Here's how the part is built. I have some questions about the finished solid (model axes, mm). Face numbers are marked on the shaded views. A direction names the side the tool comes from. Coordinates: 2 decimals unless noted, no trailing zeros. Order: outer loops, then holes, each group sorted by start corner. A loop starts at its lowest first (then second) coordinate and runs counter-clockwise, first axis right, second up.
```python
from build123d import *

# Parameters (mm, degrees)
BOSS_EXTRUDE1_DEPTH = 10
SKETCH2_R           = 1.75
CUT_EXTRUDE1_DEPTH  = 10
BOSS_EXTRUDE2_DEPTH = 5
CUT_EXTRUDE2_DEPTH  = 3
FILLET1_R           = 4
FILLET2_R           = 1.5
FILLET3_R           = 2
FILLET4_R           = 1


with BuildPart() as part:
    # Sketch1 → Boss-Extrude1 (new body)
    with BuildSketch(Plane(origin=(0, 0, 0), x_dir=(1, 0, 0), z_dir=(0, 1, 0))):
        with BuildLine():
            Line((-47.236109069, 5), (-55.236109069, 5))
            Line((-55.236109069, 5), (-55.236109069, -5))
            Line((-55.236109069, -5), (-47.236109069, -5))
            ThreePointArc((-47.236109069, -5), (-47.5, 0), (-47.236109069, 5))
        make_face()
    extrude(amount=-BOSS_EXTRUDE1_DEPTH)

    # Sketch2 → Cut-Extrude1 (cut)
    with BuildSketch(Plane.ZY.offset(55.236109069)):
        with Locations((0, -5)):
            Circle(SKETCH2_R)
    extrude(amount=-CUT_EXTRUDE1_DEPTH, mode=Mode.SUBTRACT)

    # Sketch3 → Boss-Extrude2 (add, symmetric)
    with BuildSketch(Plane.XY):
        Polygon((-80.236109069, -13), (-166.418406548, -137), (-176.418406548, -137), (-176.418406548, -145), (-162.236109069, -145), (-76.053811591, -21), (-50.236109069, -21), (-50.236109069, -10), (-55.236109069, -10), (-55.236109069, -13), align=None)
    extrude(amount=BOSS_EXTRUDE2_DEPTH, both=True)

    # Sketch4 → Cut-Extrude2 (cut)
    with BuildSketch(Plane.XY.offset(5)):
        Polygon((-164.327257809, -141), (-165.503528974, -138.75), (-79.321231496, -14.75), (-55.236109069, -14.75), (-55.236109069, -19.25), (-76.968689164, -19.25), (-163.150986643, -143.25), align=None)
    cut_extrude2 = extrude(amount=-CUT_EXTRUDE2_DEPTH, mode=Mode.SUBTRACT)

    # Mirror1: Cut-Extrude2 across plane
    add(cut_extrude2.mirror(Plane.XY), mode=Mode.SUBTRACT)

    # Fillet1
    fillet1_edges = [part.edges().sort_by_distance(p)[0] for p in [
        (-55.236109069, -13, 0),
    ]]
    fillet(fillet1_edges, radius=FILLET1_R)

    # Fillet2
    fillet2_edges = [part.edges().sort_by_distance(p)[0] for p in [
        (-50.236109069, -10, 0),
    ]]
    fillet(fillet2_edges, radius=FILLET2_R)

    # Fillet3
    fillet3_edges = [part.edges().sort_by_distance(p)[0] for p in [
        (-80.236109069, -13, 0),
        (-166.418406548, -137, 0),
        (-176.418406548, -137, 0),
        (-176.418406548, -145, 0),
        (-162.236109069, -145, 0),
        (-76.053811591, -21, 0),
        (-55.236109069, 0, 0),
    ]]
    fillet(fillet3_edges, radius=FILLET3_R)

    # Fillet4
    fillet4_edges = [part.edges().sort_by_distance(p)[0] for p in [
        (-55.236109069, -14.75, 3.5),
        (-55.236109069, -19.25, 3.5),
        (-76.968689164, -19.25, 3.5),
        (-163.150986643, -143.25, 3.5),
        (-165.503528974, -138.75, 3.5),
        (-79.321231496, -14.75, 3.5),
        (-55.236109069, -19.25, -3.5),
        (-55.236109069, -14.75, -3.5),
        (-79.321231496, -14.75, -3.5),
        (-165.503528974, -138.75, -3.5),
        (-163.150986643, -143.25, -3.5),
        (-76.968689164, -19.25, -3.5),
    ]]
    fillet(fillet4_edges, radius=FILLET4_R)


solid = part.part
```
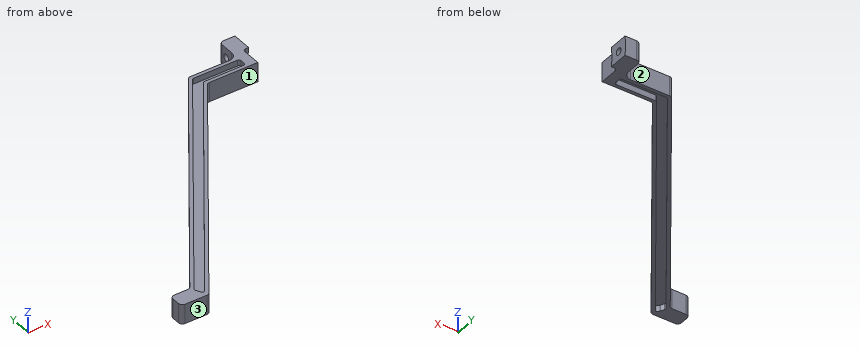
Q1. If we section it at B-B on y = -5: Write out the boundary of the cut face in (x, z).
Q2. If we section it at C-C on y = -37: Write out the boundary of the cut face in (x, z), then the cut area to 3 significant figures.
Q3. For the marked faces 1, 2 and 3, which set-ups out of +Z, -Z, +X, -X, +Y, -Y let a thin tool reach every point of the face, with its end or its side?
Q4. Will these pins go through, and if not, where does the flat tip stop? pin 1 (2.5 mm diameter, centred on x = -65, z = -3.5, fed in from +Y); pin 2 (2.5 mm diameter, centred on x = -70.5, z = -3, fed in from -Y); pin 3 (4 mm diameter, centred on y = -35.5, z = -2, fed in from +X).
Q5. If we section it at A-A on z = 0: Write out the boundary of the cut face in (x, y).
Q6. I need wall thicknesses on L1, parallel to Y at x = -53.5, z = 0; L2, parallel to Z at x = -49.75, y = -5; L3, parallel to Y at x = -170, z = -4. Which ranges of each line are inside material? Lowest first, please.
Reply:
1. outline: (-55.24, -5) - (-47.24, -5) arc R47.5 cw to (-47.47, -1.75) - (-55.24, -1.75) - close; (-55.24, 1.75) - (-47.47, 1.75) arc R47.5 cw to (-47.24, 5) - (-55.24, 5) - close
2. outline: (-96.92, -5) - (-94.79, -5) - (-94.79, -2) - (-89.31, -2) - (-89.31, -5) - (-87.17, -5) - (-87.17, 5) - (-89.31, 5) - (-89.31, 2) - (-94.79, 2) - (-94.79, 5) - (-96.92, 5) - close
2. area: 64.5 mm2
3. face 1: +Z, -Z, +X, -Y
3. face 2: +Z, -Z, -X, +Y
3. face 3: +Z, -Z, +X, -X, -Y
4. pin 1: stops at y = -13
4. pin 2: stops at y = -21
4. pin 3: stops at x = -84.74
5. outline: (-176.42, -143) arc R2 ccw to (-174.42, -145) - (-163.28, -145) arc R2 ccw to (-161.64, -144.14) - (-76.65, -21.86) arc R2 cw to (-75.01, -21) - (-50.24, -21) - (-50.24, -11.5) arc R1.5 cw to (-48.74, -10) - (-47.5, -10) - (-47.5, -6.75) - (-55.24, -6.75) - (-55.24, -9) arc R4 cw to (-59.24, -13) - (-79.19, -13) arc R2 ccw to (-80.83, -13.86) - (-165.82, -136.14) arc R2 cw to (-167.46, -137) - (-174.42, -137) arc R2 ccw to (-176.42, -139) - close; (-55.24, -3.25) - (-47.5, -3.25) - (-47.5, 0) - (-53.24, 0) arc R2 ccw to (-55.24, -2) - close
6. L1: y = -21 to -6.75, -3.25 to -0.02
6. L2: z = -5 to -1.75, 1.75 to 5
6. L3: y = -145 to -137
